```python
from build123d import *

# Parameters (mm, degrees)
F0_W     = 137.5
F0_H     = 150
F0_W_2   = 25
F1_DEPTH = 150


with BuildPart() as f1:
    # F0 (on Top) → F1 (new body)
    with BuildSketch(Plane.XY):
        with BuildLine():
            Line((200, -100), (200, 100))
            Line((200, 100), (5, 100))
            ThreePointArc((5, 100), (0, 95), (-5, 100))
            Line((-5, 100), (-200, 100))
            Line((-200, 100), (-200, -100))
            Line((-200, -100), (-5, -100))
            ThreePointArc((-5, -100), (0, -95), (5, -100))
            Line((5, -100), (200, -100))
        make_face()
        with Locations((-106.25, 0)):
            Rectangle(F0_W, F0_H, mode=Mode.SUBTRACT)
        Rectangle(F0_W_2, F0_H, mode=Mode.SUBTRACT)
        with Locations((106.25, 0)):
            Rectangle(F0_W, F0_H, mode=Mode.SUBTRACT)
    extrude(amount=F1_DEPTH)


solid = f1.part
```
The listing builds one solid part. Answer for the finished solid, in the listing's coordinates (mm). A direction names the side the tool comes from. Coordinates: 2 decimals unless noted, no trailing zeros. Write each loop counter-clockwise with the first axis right and the second up, starting at its lowest first coordinate (ties: lowest second). Pieces come first, ordered by that corner, then holes. Notation, with made-up numbers: M 71,-27.5 L 118,-27.5 A28 ccw 118,8.5 Z; hole C 32,39.25 d5. An arc over 180 degrees is marked long. Use a Markdown table: item, result. Add a question column.
1. For a pull along X with two mould halves and no side action, classify faces 1 (the flat face through (-104, -100, 74)), 2 (the flat face through (-200, 1, 74)), 3 (the flat face through (105, -75, 74)) as +X half, -X half, draft (parallel to the pull), parting line (faces both ways), or undercut.
2. Section C-C (z = 89.5) is taken. Give the vertices of the cut face in (x, y).
3. Section B-B (y = -67) is taken. Give the vertices of the cut face in (x, z), plus the area to 3 significant figures.
4. Straight lines are drawn through the part: line 1 along X through (y, z) = (5.5, 70.5); line 2 along Y through (x, z) = (-95, 34). For each, find the intervals that lie inside material, in ascending order. Write a range as [from, to].
5. Section D-D (x = 0) is taken. Give the vertices of the cut face in (y, z).
6. Which of the six approach directions +Z, -Z, +X, -X, +Y, -Y give full straight-line access (tool end or side, diameter ignored) to faces 4 (the cylindrical face through (0, 95, 74)), 5 (the flat face through (-107, 75, 74))?
7. Section A-A (x = -171) is taken. Give the vertices of the cut face in (y, z), plus the area to 3 significant figures.
Data:
| question | item | result |
|---|---|---|
| 1 | face 1 | draft |
| 1 | face 2 | -X half |
| 1 | face 3 | undercut |
| 2 | outline | M -200,-100 L -5,-100 A5 cw 5,-100 L 200,-100 L 200,100 L 5,100 A5 cw -5,100 L -200,100 Z; hole M -175,-75 L -37.5,-75 L -37.5,75 L -175,75 Z; hole M -12.5,-75 L 12.5,-75 L 12.5,75 L -12.5,75 Z; hole M 37.5,-75 L 175,-75 L 175,75 L 37.5,75 Z |
| 3 | outline | M -200,0 L -175,0 L -175,150 L -200,150 Z; M -37.5,0 L -12.5,0 L -12.5,150 L -37.5,150 Z; M 12.5,0 L 37.5,0 L 37.5,150 L 12.5,150 Z; M 175,0 L 200,0 L 200,150 L 175,150 Z |
| 3 | area | 15,000 mm2 |
| 4 | line 1 | x = [-200, -175], [-37.5, -12.5], [12.5, 37.5], [175, 200] |
| 4 | line 2 | y = [-100, -75], [75, 100] |
| 5 | outline | M -95,0 L -75,0 L -75,150 L -95,150 Z; M 75,0 L 95,0 L 95,150 L 75,150 Z |
| 6 | face 4 | +Z, -Z, +Y |
| 6 | face 5 | +Z, -Z |
| 7 | outline | M -100,0 L -75,0 L -75,150 L -100,150 Z; M 75,0 L 100,0 L 100,150 L 75,150 Z |
| 7 | area | 7,500 mm2 |
